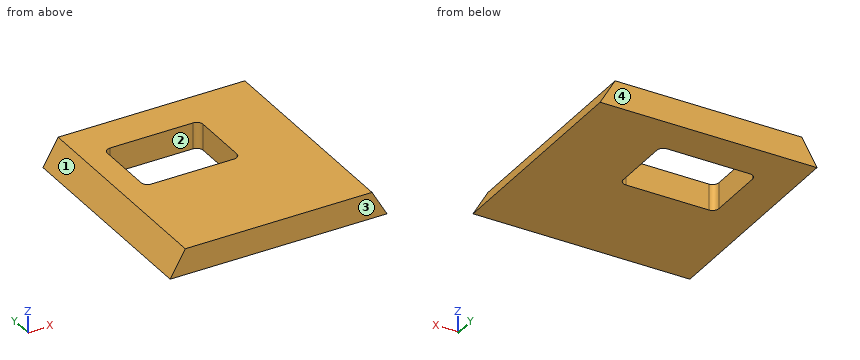
Autodesk Inventor part; units mm, degrees
ref_plane "YZ Plane" through (0, 0, 0) normal (1, 0, 0) x (0, 1, 0)
ref_plane "XZ Plane" through (0, 0, 0) normal (0, 1, 0) x (-1, 0, 0)
ref_plane "XY Plane" through (0, 0, 0) normal (0, 0, 1) x (1, 0, 0)
sketch "Sketch1" plane through (0, 0, 0) normal (0, 1, 0) x (-1, 0, 0)
  line L0 (-107.95, -0.0035) -> (-53.978, 93.4857)
  line L1 (-53.978, 93.4857) -> (53.972, 93.4892)
  line L2 (53.972, 93.4892) -> (107.95, 0.0035)
  line L3 (107.95, 0.0035) -> (53.978, -93.4857)
  line L4 (53.978, -93.4857) -> (-53.972, -93.4892)
  line L5 (-53.972, -93.4892) -> (-107.95, -0.0035)
  line L6 (-92.964, 0.0336) -> (-46.4529, 80.526)
  line L7 (-46.4529, 80.526) -> (46.5111, 80.4924)
  line L8 (46.5111, 80.4924) -> (92.964, -0.0336)
  line L9 (92.964, -0.0336) -> (46.4529, -80.526)
  line L10 (46.4529, -80.526) -> (-46.5111, -80.4924)
  line L11 (-46.5111, -80.4924) -> (-92.964, 0.0336)
  line L12 (53.978, -93.4857) -> (46.4529, -80.526)
  line L13 (-53.972, -93.4892) -> (-46.5111, -80.4924)
  point P0 (0, 0)
  point P1 (0, 0)
  point P2 (0, 0)
  point P3 (0, 0)
  dimension "d0" = 215.9
  dimension "d1" = 14.986
extrude "Extrusion1" add sketch "Sketch1" along normal blind 107.95 contours L13 L10 L12 L4
sketch "Sketch2" plane through (53.972, 0, -93.4892) normal (0, 0, -1) x (-1, 0, 0)
  line L0 (85.725, 88.9) -> (44.45, 88.9)
  line L1 (41.275, 85.725) -> (41.275, 57.15)
  line L2 (44.45, 53.975) -> (85.725, 53.975)
  line L3 (88.9, 57.15) -> (88.9, 85.725)
  line L4 (107.95, 0) -> (107.95, 107.95)
  line L5 (0, 107.95) -> (107.95, 107.95)
  arc A0 (44.45, 88.9) -> (41.275, 85.725) centre (44.45, 85.725) ccw
  arc A1 (88.9, 85.725) -> (85.725, 88.9) centre (85.725, 85.725) ccw
  arc A2 (41.275, 57.15) -> (44.45, 53.975) centre (44.45, 57.15) ccw
  arc A3 (85.725, 53.975) -> (88.9, 57.15) centre (85.725, 57.15) ccw
  point P0 (53.975, 0)
  point P1 (41.275, 53.975)
  point P2 (41.275, 88.9)
  point P3 (88.9, 53.975)
  dimension "d4" = 47.625
  dimension "d5" = 34.925
  dimension "d6" = 19.05
  dimension "d7" = 19.05
  dimension "d8" = 3.175
extrude "Extrusion2" cut sketch "Sketch2" against normal up to surface (12.9994 mm away)
properties part number "SatelliteSideWallCamera_v2"
Input: part model. Units: mm. Frame: model coordinates. Face numbers are marked on the shaded views. Round coordinates to 2 decimals unless told otherwise and drop trailing zeros. Loops run counter-clockwise (first coordinate to the right, second up) from the corner with the lowest first, then second, coordinate; pieces in that order, holes last. Notation, with made-up numbers: (-11.5, 36.25) -> (14.5, 36.25) arc R16 cw to (14.5, 52.25) -> close; hole circle Ø6 at (-39, 58.5). An arc over 180 degrees is marked (long way). Answer as a JSON object with one key per item and string values. Group by question number.
1) Section query B-B on x = -33.5. Output: boundary loops of the cut face in (y, z).
2) Draft query along Y for the marked faces 1, 2, 3 and 4. Return one class per face: +Y half, -Y half, draft (parallel to the pull), parting line (faces both ways), or undercut.
3) Section query A-A on y = 76. Output: boundary loops of the cut face in (x, z).
4) Ray query, L1, parallel to Y at x = 7, z = -89 (3 decimals); L2, parallel to Z at x = 34.5, y = 43; L3, parallel to Y at x = 11, z = -84.75 (3 decimals). Return the intervals inside material, ascending.
5) Pin query (flat end, axial travel): pin 1 (3 mm diameter, centred on y = 88.5, z = -85, fed in from -X); pin 2 (2 mm diameter, centred on y = 17.5, z = -86, fed in from +X); pin 3 (4 mm diameter, centred on x = -2, z = -86, fed in from -Y); pin 4 (1.5 mm diameter, centred on y = 46.5, z = -85, fed in from -X). Return the tip coordinate at first contact, or that it passes through.
6) Section query D-D on z = -92. Output: boundary loops of the cut face in (x, y) (3 decimals).
7) Section query C-C on z = -82.5. Output: boundary loops of the cut face in (x, y) (3 decimals), plus the area to 3 significant figures.
Reply:
{
 "1": {"outline": "(0, -93.49) -> (54.5, -93.49) -> (54.5, -80.52) -> (0, -80.52) -> close; (88.38, -93.49) -> (107.95, -93.49) -> (107.95, -80.52) -> (88.38, -80.52) -> close"},
 "2": {"face 1": "draft", "face 2": "undercut", "face 3": "-Y half", "face 4": "+Y half"},
 "3": {"outline": "(-53.98, -93.49) -> (-34.93, -93.49) -> (-34.93, -80.52) -> (-46.45, -80.53) -> close; (12.7, -93.49) -> (53.97, -93.49) -> (46.51, -80.49) -> (12.7, -80.5) -> close"},
 "4": {"L1": "y = 0 to 53.975, 88.9 to 107.95", "L2": "z = -93.49 to -80.5", "L3": "y = 0 to 54.34, 88.535 to 107.95"},
 "5": {"pin 1": "stops at x = -49.92", "pin 2": "stops at x = 50.25", "pin 3": "stops at y = 0", "pin 4": "stops at x = -49.49"},
 "6": {"outline": "(-53.115, 0) -> (53.117, 0) -> (53.117, 107.95) -> (-53.115, 107.95) -> close; hole (-34.928, 57.15) arc R3.175 ccw to (-31.753, 53.975) -> (9.522, 53.975) arc R3.175 ccw to (12.697, 57.15) -> (12.697, 85.725) arc R3.175 ccw to (9.522, 88.9) -> (-31.753, 88.9) arc R3.175 ccw to (-34.928, 85.725) -> close"},
 "7": {"outline": "(-47.599, 0) -> (47.664, 0) -> (47.664, 107.95) -> (-47.599, 107.95) -> close; hole (-34.928, 57.15) arc R3.175 ccw to (-31.753, 53.975) -> (9.522, 53.975) arc R3.175 ccw to (12.697, 57.15) -> (12.697, 85.725) arc R3.175 ccw to (9.522, 88.9) -> (-31.753, 88.9) arc R3.175 ccw to (-34.928, 85.725) -> close", "area": "8,630 mm2"}
}
